```python
from build123d import *

# Parameters (mm, degrees)
F1_DEPTH = 3.175


# Not quite as in the source:
# - a length typed as a fraction of an inch, garbled in the dataset ("3 / 203.2 mm" for 3/8 in), is restored


with BuildPart() as f1:
    # F0 (on Front) → F1 (new body)
    with BuildSketch(Plane.XZ):
        Polygon((-178.9622853069, -44.2643848114), (-153.5622853069, -44.2643848114), (-153.5622853069, -47.4393848114), (-128.1622853069, -47.4393848114), (-128.1622853069, -44.2643848114), (-102.7622853069, -44.2643848114), (-102.7622853069, -47.4393848114), (-77.3622853069, -47.4393848114), (-77.3622853069, -44.2643848114), (-51.9622853069, -44.2643848114), (-51.9622853069, -47.4393848114), (-26.5622853069, -47.4393848114), (-26.5622853069, -44.2643848114), (-26.5622853069, 108.1356151886), (-26.5622853069, 111.3106151886), (-51.9622853069, 111.3106151886), (-51.9622853069, 108.1356151886), (-77.3622853069, 108.1356151886), (-77.3622853069, 111.3106151886), (-102.7622853069, 111.3106151886), (-102.7622853069, 108.1356151886), (-128.1622853069, 108.1356151886), (-128.1622853069, 111.3106151886), (-153.5622853069, 111.3106151886), (-153.5622853069, 108.1356151886), (-178.9622853069, 108.1356151886), (-178.9622853069, 82.7356151886), (-182.1372853069, 82.7356151886), (-182.1372853069, 57.3356151886), (-178.9622853069, 57.3356151886), (-178.9622853069, 31.9356151886), (-182.1372853069, 31.9356151886), (-182.1372853069, 6.5356151886), (-178.9622853069, 6.5356151886), (-178.9622853069, -18.8643848114), (-182.1372853069, -18.8643848114), (-182.1372853069, -44.2643848114), (-182.1372853069, -47.4393848114), (-178.9622853069, -47.4393848114), align=None)
        Polygon((-26.5622853069, 108.1356151886), (-26.5622853069, -44.2643848114), (-1.1622853069, -44.2643848114), (-1.1622853069, -47.4393848114), (24.2377146931, -47.4393848114), (24.2377146931, -44.2643848114), (49.6377146931, -44.2643848114), (49.6377146931, -47.4393848114), (75.0377146931, -47.4393848114), (75.0377146931, -44.2643848114), (100.4377146931, -44.2643848114), (100.4377146931, -47.4393848114), (125.8377146931, -47.4393848114), (129.0127146931, -47.4393848114), (129.0127146931, -44.2643848114), (129.0127146931, -18.8643848114), (125.8377146931, -18.8643848114), (125.8377146931, 6.5356151886), (129.0127146931, 6.5356151886), (129.0127146931, 31.9356151886), (125.8377146931, 31.9356151886), (125.8377146931, 57.3356151886), (129.0127146931, 57.3356151886), (129.0127146931, 82.7356151886), (125.8377146931, 82.7356151886), (125.8377146931, 108.1356151886), (125.8377146931, 111.3106151886), (100.4377146931, 111.3106151886), (100.4377146931, 108.1356151886), (75.0377146931, 108.1356151886), (75.0377146931, 111.3106151886), (49.6377146931, 111.3106151886), (49.6377146931, 108.1356151886), (24.2377146931, 108.1356151886), (24.2377146931, 111.3106151886), (-1.1622853069, 111.3106151886), (-1.1622853069, 108.1356151886), align=None)
    extrude(amount=F1_DEPTH)


solid = f1.part
```
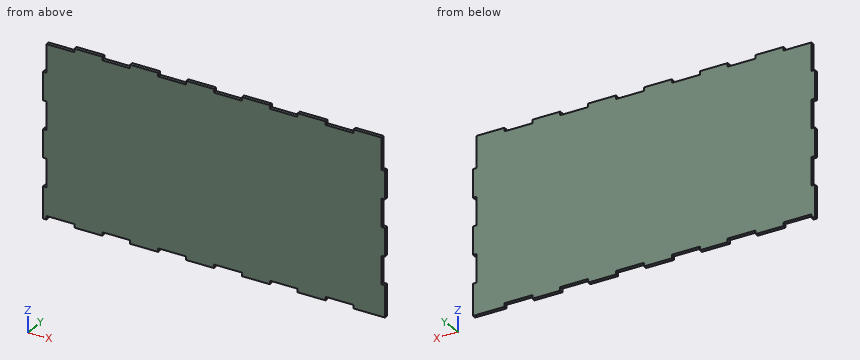
Verification items for the finished model (mm, model axes). Give positions to 0.01 mm unless a question says otherwise; leave off trailing zeros. Order: outer loops, then holes, each group sorted by start corner. A loop starts at its lowest first (then second) coordinate and runs counter-clockwise, first axis right, second up. Notation, with made-up numbers: (42.25, -17) - (48.25, -17) arc R24 ccw to (48.25, 1) - close; hole circle Ø8 at (59, 37). An arc over 180 degrees is marked (long way). Answer as CSV lines item,"result". Start each with the question number.
Item 1: Section check B-B, the plane x = 79. Record the boundary of the cut face in (y, z) (3 decimals).
Item 2: Gauge pin test, flat ends, axial feed: pin 1 (1.6 mm diameter, centred on x = -171.5, y = -1.5, fed in from +Z); pin 2 (1.6 mm diameter, centred on y = -2, z = 109, fed in from +X); pin 3 (1.6 mm diameter, centred on y = -2, z = -11.5, fed in from -X). Record the tip position at first contact, or that the pin passes through.
Item 3: Section check A-A, the plane z = -7.5. Record the boundary of the cut face in (x, y) (3 decimals).
Item 4: Material ranges on L1, parallel to Z at x = -12.5, y = -2.2; L2, parallel to X at y = -0.7, z = 87, recorded low to high.
Filled in:
1,outline,"(-3.175, -44.264) - (0, -44.264) - (0, 108.136) - (-3.175, 108.136) - close"
2,pin 1,"z = 108.14"
2,pin 2,"x = 125.84"
2,pin 3,"x = -178.96"
3,outline,"(-178.962, -3.175) - (125.838, -3.175) - (125.838, 0) - (-178.962, 0) - close"
4,L1,"-44.26 to 108.14"
4,L2,"-178.96 to 125.84"
